Could you check a few things on this model? Use its own coordinates, in mm. A direction names the side the tool comes from. Coordinates: 2 decimals unless noted, no trailing zeros. Loops run counter-clockwise (first coordinate to the right, second up) from the corner with the lowest first, then second, coordinate; pieces in that order, holes last. Notation, with made-up numbers: M -39,24.5 L 6,24.5 A14 cw 6,40.5 Z; hole C 49,-9.75 d7. An arc over 180 degrees is marked long. Return JSON: item names as keys, results as strings. Group by question number.
from build123d import *

# Parameters (mm, degrees)
F1_DEPTH  = 25
F3_W      = 2
F3_H      = 15
F3_W_2    = 5.2175602431
F4_DEPTH  = 14
F5_W      = 6.9340183245
F5_H      = 15
F5_W_2    = 2
F6_DEPTH  = 14
F7_R      = 10
F8_DEPTH  = 15
F10_DEPTH = 10


with BuildPart() as f1:
    # F0 (on Front) → F1 (new body)
    with BuildSketch(Plane.XZ):
        Polygon((10, -28), (24, -28), (24, -20), (15, 0), (-15, 0), (-24, -20), (-24, -28), (-10, -28), (-5, -18), (5, -18), align=None)
    extrude(amount=F1_DEPTH)

    # F3 (on face) → F4 (cut)
    with BuildSketch(Plane.XY):
        with Locations((-14, -12.5)):
            Rectangle(F3_W, F3_H)
        with Locations((-17.6087801216, -12.5)):
            Rectangle(F3_W_2, F3_H)
    extrude(amount=-F4_DEPTH, mode=Mode.SUBTRACT)

    # F5 (on face) → F6 (cut)
    with BuildSketch(Plane.XY):
        with Locations((18.4670091623, -12.5)):
            Rectangle(F5_W, F5_H)
        with Locations((14, -12.5)):
            Rectangle(F5_W_2, F5_H)
    extrude(amount=-F6_DEPTH, mode=Mode.SUBTRACT)

    # F7 (on face) → F8 (join)
    with BuildSketch(Plane.XY):
        with Locations((0, -12.5)):
            Circle(F7_R)
    extrude(amount=F8_DEPTH)

    # F9 (on face) → F10 (cut)
    with BuildSketch(Plane.XY.offset(15)):
        with BuildLine():
            Line((9.1950891808, -8.5693085904), (-9.1950891808, -8.5693085904))
            ThreePointArc((-9.1950891808, -8.5693085904), (-9.79670587, -10.4938708676), (-10, -12.5))
            ThreePointArc((-10, -12.5), (-9.7812549358, -14.5801566962), (-9.1345896238, -16.5693085904))
            Line((-9.1345896238, -16.5693085904), (9.1345896238, -16.5693085904))
            ThreePointArc((9.1345896238, -16.5693085904), (9.7812549358, -14.5801566962), (10, -12.5))
            ThreePointArc((10, -12.5), (9.79670587, -10.4938708676), (9.1950891808, -8.5693085904))
        make_face()
        with BuildLine():
            Line((10, -8.5693085904), (9.1950891808, -8.5693085904))
            ThreePointArc((9.1950891808, -8.5693085904), (9.79670587, -10.4938708676), (10, -12.5))
            Line((10, -12.5), (10, -8.5693085904))
        make_face()
    extrude(amount=-F10_DEPTH, mode=Mode.SUBTRACT)


solid = f1.part
(1) Imagine slicing it at D-D, the plane x = -6. Write out the boundary of the cut face in (y, z).
(2) Will these pins go through, and if not, where does the flat tip stop? P1, Ø6, axis at x = -17, z = -9.5, coming from the +Y side; P2, Ø11, axis at y = -11, z = -7.5, coming from the -X side; P3, Ø3, axis at x = 1, y = -11, coming from the -Z side; P4, Ø3, axis at x = 15.5, y = -3, coming from the +Z side.
(3) We'd pull the mould along X, two halves only. Please class faces 4 (the face through (13, -13, -7)), 5 (the face through (17, -12, -28)), 6 (the face through (-20.218, -13, -13)): +X half, -X half, draft (parallel to the pull), parting line (faces both ways), or undercut.
(4) For faces 1 (the face through (-16, -20, -8)), 2 (the face through (0, -12, -18)), 3 (the face through (16, -5, -8)), which set-ups out of +Z, -Z, +X, -X, +Y, -Y let a thin tool reach every point of the face, with its end or its side?
(5) Imagine slicing it at A-A, the plane z = 11. Write out the boundary of the cut face in (x, y).
(6) Imagine slicing it at C-C, the plane y = -12.5. Write out the boundary of the cut face in (x, z), then the cut area to 3 significant figures.
(7) If I drill on L1, parallel to X at y = -6.75, z = -11; L2, parallel to Z at x = 10.5, y = -21.25; L3, parallel to Z at x = 4.5, y = -9.5, over which ranges is the centre line in solid material (lowest first)? Write a range as [from, to].
(8) Imagine slicing it at B-B, the plane x = 0. Write out the boundary of the cut face in (y, z).
Checks:
{
 "1": {"outline": "M -25,-20 L 0,-20 L 0,0 L -4.5,0 L -4.5,15 L -8.57,15 L -8.57,5 L -16.57,5 L -16.57,15 L -20.5,15 L -20.5,0 L -25,0 Z"},
 "2": {"P1": "y = 0", "P2": "x = -20.85", "P3": "z = -18", "P4": "z = 0"},
 "3": {"face 4": "+X half", "face 5": "draft", "face 6": "undercut"},
 "4": {"face 1": "+Z", "face 2": "-Z, +Y, -Y", "face 3": "+Z, +X"},
 "5": {"outline": "M -9.2,-8.57 L 9.2,-8.57 A10 ccw Z; M -9.13,-16.57 A10 ccw 9.13,-16.57 Z"},
 "6": {"outline": "M -24,-28 L -10,-28 L -5,-18 L 5,-18 L 10,-28 L 24,-28 L 24,-20 L 21.3,-14 L 13,-14 L 13,0 L 10,0 L 10,5 L -10,5 L -10,0 L -13,0 L -13,-14 L -20.22,-14 L -20.22,-11.59 L -24,-20 Z", "area": "971 mm²"},
 "7": {"L1": "[-13, 13]", "L2": "[-28, 0]", "L3": "[-18, 5]"},
 "8": {"outline": "M -25,-18 L 0,-18 L 0,0 L -2.5,0 L -2.5,15 L -8.57,15 L -8.57,5 L -16.57,5 L -16.57,15 L -22.5,15 L -22.5,0 L -25,0 Z"}
}
